For this review, take the finished solid that the model builds, in its own axes (mm). A direction names the side the tool comes from. Coordinates: 2 decimals unless noted, no trailing zeros. One line per item, written item: value.
from build123d import *

# Parameters (mm, degrees)
ESQUISSE1_R                  = 8
BOSS_EXTRU_1_DEPTH           = 16
ENL_V_MAT_EXTRU_1_DEPTH      = 10
ESQUISSE3_R                  = 5
ENL_V_MAT_EXTRU_2_DEPTH      = 20.595917942
R_P_TITION_CIRCULAIRE1_COUNT = 10
CONG_1_R                     = 1
CONG_2_R                     = 1
BOSS_EXTRU_2_DEPTH           = 2
ESQUISSE5_R                  = 3.4
ENL_V_MAT_EXTRU_3_DEPTH      = 3.5
ESQUISSE6_R                  = 0.5
ENL_V_MAT_EXTRU_4_DEPTH      = 6.5
CONG_3_R                     = 2


# Some blends are built 0.0001 mm under size
with BuildPart() as part:
    # Esquisse1 → Boss.-Extru.1 (new body)
    with BuildSketch(Plane(origin=(0, 0, 0), x_dir=(1, 0, 0), z_dir=(0, 1, 0))):
        with Locations(Location((0, 0, 0), (0, 0, 270))):
            Circle(ESQUISSE1_R)
    extrude(amount=BOSS_EXTRU_1_DEPTH)

    # Esquisse2 → Enlèv. mat.-Extru.1 (cut)
    with BuildSketch(Plane(origin=(0, 16, 0), x_dir=(1, 0, 0), z_dir=(0, 1, 0))):
        with BuildLine():
            ThreePointArc((0, 3.15), (-2.720753572, 1.587450787), (-2.74226184, -1.55))
            Line((-2.74226184, -1.55), (0, -1.55))
            Line((0, -1.55), (0, 3.15))
        make_face()
        with BuildLine():
            Line((0, 3.15), (0, -1.55))
            Line((0, -1.55), (2.74226184, -1.55))
            ThreePointArc((2.74226184, -1.55), (3.046360517, -0.801366085), (3.15, 0))
            ThreePointArc((3.15, 0), (2.227386361, 2.227386361), (0, 3.15))
        make_face()
    extrude(amount=-ENL_V_MAT_EXTRU_1_DEPTH, mode=Mode.SUBTRACT)

    # Esquisse3 → Enlèv. mat.-Extru.2 (cut, through all)
    with BuildSketch(Plane(origin=(0, 16, 0), x_dir=(1, 0, 0), z_dir=(0, 1, 0))):
        with Locations((0, 12.5)):
            Circle(ESQUISSE3_R)
    enl_v_mat_extru_2 = extrude(amount=-ENL_V_MAT_EXTRU_2_DEPTH, mode=Mode.SUBTRACT)

    # Répétition circulaire1: Enlèv. mat.-Extru.2 ×10 about axis
    r_p_tition_circulaire1_axis = Axis((0, 0, 0), (0, 1, 0))
    for i in range(1, R_P_TITION_CIRCULAIRE1_COUNT):
        add(enl_v_mat_extru_2.rotate(r_p_tition_circulaire1_axis, i * 360 / R_P_TITION_CIRCULAIRE1_COUNT), mode=Mode.SUBTRACT)

    # Congé1
    cong_1_edges = [part.edges().sort_by_distance(p)[0] for p in [
        (1.733176275, 8, -7.81),
        (-1.733176275, 8, -7.81),
        (-3.18843376, 8, -7.33715818),
        (-5.992771881, 8, -5.299687272),
        (-6.892170469, 8, -4.061771316),
        (-7.963332315, 8, -0.765074136),
        (-1.733176275, 8, 7.81),
        (1.733176275, 8, 7.81),
        (-7.963332315, 8, 0.765074136),
        (-6.892170469, 8, 4.061771316),
        (-5.992771881, 8, 5.299687272),
        (-3.18843376, 8, 7.33715818),
        (3.18843376, 8, 7.33715818),
        (5.992771881, 8, 5.299687272),
        (6.892170469, 8, 4.061771316),
        (7.963332315, 8, 0.765074136),
        (7.963332315, 8, -0.765074136),
        (6.892170469, 8, -4.061771316),
        (5.992771881, 8, -5.299687272),
        (3.18843376, 8, -7.33715818),
    ]]
    fillet(cong_1_edges, radius=CONG_1_R)

    # Congé2
    cong_2_edges = [part.edges().sort_by_distance(p)[0] for p in [
        (-2.472135955, 0, -7.60845213),
        (-6.472135955, 0, -4.702282018),
        (-4.408389392, 0, -6.067627458),
        (0, 0, -7.5),
        (2.472135955, 0, -7.60845213),
        (4.408389392, 0, -6.067627458),
        (6.472135955, 0, -4.702282018),
        (7.132923872, 0, -2.317627458),
        (8, 0, 0),
        (7.132923872, 0, 2.317627458),
        (6.472135955, 0, 4.702282018),
        (4.408389392, 0, 6.067627458),
        (2.472135955, 0, 7.60845213),
        (0, 0, 7.5),
        (-2.472135955, 0, 7.60845213),
        (-4.408389392, 0, 6.067627458),
        (-6.472135955, 0, 4.702282018),
        (-7.132923872, 0, 2.317627458),
        (-8, 0, 0),
        (-7.132923872, 0, -2.317627458),
        (-6.846351136, 0, -4.072559992),
        (-5.988873569, 0, -5.252776613),
        (-3.145023717, 0, -7.318954474),
        (-7.932605121, 0, -0.729413986),
        (-7.932605121, 0, 0.729413986),
        (-6.846351136, 0, 4.072559992),
        (-5.988873569, 0, 5.252776613),
        (-3.145023717, 0, 7.318954474),
        (-1.757595867, 0, 7.769757109),
        (1.757595867, 0, 7.769757109),
        (3.145023717, 0, 7.318954474),
        (5.988873569, 0, 5.252776613),
        (6.846351136, 0, 4.072559992),
        (7.932605121, 0, 0.729413986),
        (7.932605121, 0, -0.729413986),
        (6.846351136, 0, -4.072559992),
        (5.988873569, 0, -5.252776613),
        (3.145023717, 0, -7.318954474),
        (1.757595867, 0, -7.769757109),
        (-1.757595867, 0, -7.769757109),
    ]]
    fillet(cong_2_edges, radius=CONG_2_R - 0.0001)  # a hair under: the kernel refuses the full size

    # Esquisse4 → Boss.-Extru.2 (add)
    with BuildSketch(Plane(origin=(0, 16, 0), x_dir=(1, 0, 0), z_dir=(0, 1, 0))):
        with BuildLine():
            ThreePointArc((-1.483028995, 7.725), (0, 7.5), (1.483028995, 7.725))
            ThreePointArc((1.483028995, 7.725), (1.757595867, 7.769757113), (2.033868336, 7.737142857))
            ThreePointArc((2.033868336, 7.737142857), (2.472135955, 7.60845213), (2.902344418, 7.454957872))
            ThreePointArc((2.902344418, 7.454957872), (3.145023719, 7.318954477), (3.340845414, 7.121358854))
            ThreePointArc((3.340845414, 7.121358854), (4.408389392, 6.067627458), (5.740436734, 5.37795371))
            ThreePointArc((5.740436734, 5.37795371), (5.988873571, 5.252776617), (6.193212514, 5.064002246))
            ThreePointArc((6.193212514, 5.064002246), (6.472135955, 4.702282018), (6.729960252, 4.325232365))
            ThreePointArc((6.729960252, 4.325232365), (6.84635114, 4.072559993), (6.888630426, 3.797600671))
            ThreePointArc((6.888630426, 3.797600671), (7.132923872, 2.317627458), (7.805192751, 0.976711892))
            ThreePointArc((7.805192751, 0.976711892), (7.932605125, 0.729413987), (7.986960012, 0.456584897))
            ThreePointArc((7.986960012, 0.456584897), (8, 0), (7.986960012, -0.456584897))
            ThreePointArc((7.986960012, -0.456584897), (7.932605125, -0.729413987), (7.805192751, -0.976711892))
            ThreePointArc((7.805192751, -0.976711892), (7.132923872, -2.317627458), (6.888630426, -3.797600671))
            ThreePointArc((6.888630426, -3.797600671), (6.84635114, -4.072559993), (6.729960252, -4.325232365))
            ThreePointArc((6.729960252, -4.325232365), (6.472135955, -4.702282018), (6.193212514, -5.064002246))
            ThreePointArc((6.193212514, -5.064002246), (5.988873571, -5.252776617), (5.740436734, -5.37795371))
            ThreePointArc((5.740436734, -5.37795371), (4.408389392, -6.067627458), (3.340845414, -7.121358854))
            ThreePointArc((3.340845414, -7.121358854), (3.145023719, -7.318954477), (2.902344418, -7.454957872))
            ThreePointArc((2.902344418, -7.454957872), (2.472135955, -7.60845213), (2.033868336, -7.737142857))
            ThreePointArc((2.033868336, -7.737142857), (1.757595867, -7.769757113), (1.483028995, -7.725))
            ThreePointArc((1.483028995, -7.725), (0, -7.5), (-1.483028995, -7.725))
            ThreePointArc((-1.483028995, -7.725), (-1.757595867, -7.769757113), (-2.033868336, -7.737142857))
            ThreePointArc((-2.033868336, -7.737142857), (-2.472135955, -7.60845213), (-2.902344418, -7.454957872))
            ThreePointArc((-2.902344418, -7.454957872), (-3.145023719, -7.318954477), (-3.340845414, -7.121358854))
            ThreePointArc((-3.340845414, -7.121358854), (-4.408389392, -6.067627458), (-5.740436734, -5.37795371))
            ThreePointArc((-5.740436734, -5.37795371), (-5.988873571, -5.252776617), (-6.193212514, -5.064002246))
            ThreePointArc((-6.193212514, -5.064002246), (-6.472135955, -4.702282018), (-6.729960252, -4.325232365))
            ThreePointArc((-6.729960252, -4.325232365), (-6.84635114, -4.072559993), (-6.888630426, -3.797600671))
            ThreePointArc((-6.888630426, -3.797600671), (-7.132923872, -2.317627458), (-7.805192751, -0.976711892))
            ThreePointArc((-7.805192751, -0.976711892), (-7.932605125, -0.729413987), (-7.986960012, -0.456584897))
            ThreePointArc((-7.986960012, -0.456584897), (-8, 0), (-7.986960012, 0.456584897))
            ThreePointArc((-7.986960012, 0.456584897), (-7.932605125, 0.729413987), (-7.805192751, 0.976711892))
            ThreePointArc((-7.805192751, 0.976711892), (-7.132923872, 2.317627458), (-6.888630426, 3.797600671))
            ThreePointArc((-6.888630426, 3.797600671), (-6.84635114, 4.072559993), (-6.729960252, 4.325232365))
            ThreePointArc((-6.729960252, 4.325232365), (-6.472135955, 4.702282018), (-6.193212514, 5.064002246))
            ThreePointArc((-6.193212514, 5.064002246), (-5.988873571, 5.252776617), (-5.740436734, 5.37795371))
            ThreePointArc((-5.740436734, 5.37795371), (-4.408389392, 6.067627458), (-3.340845414, 7.121358854))
            ThreePointArc((-3.340845414, 7.121358854), (-3.145023719, 7.318954477), (-2.902344418, 7.454957872))
            ThreePointArc((-2.902344418, 7.454957872), (-2.472135955, 7.60845213), (-2.033868336, 7.737142857))
            ThreePointArc((-2.033868336, 7.737142857), (-1.757595867, 7.769757113), (-1.483028995, 7.725))
        make_face()
        with BuildLine():
            ThreePointArc((-6.98859001, 0.399511784), (-6.181867356, 2.008610463), (-5.88871522, 3.784578319))
            ThreePointArc((-5.88871522, 3.784578319), (-5.663118961, 4.114496766), (-5.41906095, 4.431001966))
            ThreePointArc((-5.41906095, 4.431001966), (-3.82060414, 5.258610463), (-2.539551366, 6.523088138))
            ThreePointArc((-2.539551366, 6.523088138), (-2.163118961, 6.657395614), (-1.779634794, 6.77))
            ThreePointArc((-1.779634794, 6.77), (0, 6.5), (1.779634794, 6.77))
            ThreePointArc((1.779634794, 6.77), (2.163118961, 6.657395614), (2.539551366, 6.523088138))
            ThreePointArc((2.539551366, 6.523088138), (3.82060414, 5.258610463), (5.41906095, 4.431001966))
            ThreePointArc((5.41906095, 4.431001966), (5.663118961, 4.114496766), (5.88871522, 3.784578319))
            ThreePointArc((5.88871522, 3.784578319), (6.181867356, 2.008610463), (6.98859001, 0.399511784))
            ThreePointArc((6.98859001, 0.399511784), (7, 0), (6.98859001, -0.399511784))
            ThreePointArc((6.98859001, -0.399511784), (6.181867356, -2.008610463), (5.88871522, -3.784578319))
            ThreePointArc((5.88871522, -3.784578319), (5.663118961, -4.114496766), (5.41906095, -4.431001966))
            ThreePointArc((5.41906095, -4.431001966), (3.82060414, -5.258610463), (2.539551366, -6.523088138))
            ThreePointArc((2.539551366, -6.523088138), (2.163118961, -6.657395614), (1.779634794, -6.77))
            ThreePointArc((1.779634794, -6.77), (0, -6.5), (-1.779634794, -6.77))
            ThreePointArc((-1.779634794, -6.77), (-2.163118961, -6.657395614), (-2.539551366, -6.523088138))
            ThreePointArc((-2.539551366, -6.523088138), (-3.82060414, -5.258610463), (-5.41906095, -4.431001966))
            ThreePointArc((-5.41906095, -4.431001966), (-5.663118961, -4.114496766), (-5.88871522, -3.784578319))
            ThreePointArc((-5.88871522, -3.784578319), (-6.181867356, -2.008610463), (-6.98859001, -0.399511784))
            ThreePointArc((-6.98859001, -0.399511784), (-7, 0), (-6.98859001, 0.399511784))
        make_face(mode=Mode.SUBTRACT)
    extrude(amount=BOSS_EXTRU_2_DEPTH)

    # Esquisse5 → Enlèv. mat.-Extru.3 (cut)
    with BuildSketch(Plane(origin=(0, 16, 0), x_dir=(1, 0, 0), z_dir=(0, 1, 0))):
        with Locations(Location((0, 0, 0), (0, 0, 270))):
            Circle(ESQUISSE5_R)
    extrude(amount=-ENL_V_MAT_EXTRU_3_DEPTH, mode=Mode.SUBTRACT)

    # Esquisse6 → Enlèv. mat.-Extru.4 (cut)
    with BuildSketch(Plane(origin=(0, 12.5, 0), x_dir=(1, 0, 0), z_dir=(0, 1, 0))):
        with Locations((0, -1.55)):
            Circle(ESQUISSE6_R)
    extrude(amount=-ENL_V_MAT_EXTRU_4_DEPTH, mode=Mode.SUBTRACT)

    # Congé3
    # the kernel refuses this fillet: 2 mm, written as the material it takes off along each edge
    with BuildSketch(Plane(origin=(-0.5, 6, 1.55), x_dir=(-1, 0, 0), z_dir=(0, 1, 0))) as cong_3_piece_1:
        with BuildLine():
            CenterArc((1, 2), CONG_3_R, 233.130102354, 36.869897646)
            ThreePointArc((-0.2, 0.4), (-0.052786405, 0.223606798), (0, 0))
            Line((0, 0), (1, 0))
        make_face()
    extrude(amount=9, mode=Mode.SUBTRACT)
    with BuildSketch(Plane(origin=(0.5, 15, 1.55), x_dir=(-0.4472135954998809, 0, 0.8944271909999544), z_dir=(0, -1, 0))) as cong_3_piece_2:
        with BuildLine():
            CenterArc((1.341640786, -1.788854382), CONG_3_R, 116.565051177, 36.869897646)
            Line((-0.447213596, -0.894427191), (0, 0))
            ThreePointArc((0, 0), (0.223606798, -0.052786405), (0.447213595, 0))
        make_face()
    extrude(amount=9, mode=Mode.SUBTRACT)


solid = part.part
1. To check wall thickness, follow probe 1 along X at (y, z) = (14.75, 0); probe 2 along X at (y, z) = (10.75, 3.75); probe 3 along Y at (x, z) = (-5, 2). State the ranges of each line that lie inside material, in increasing order. Write a range as from..to.
Return value:
probe 1: x = -8..-3.4, 3.4..8
probe 2: x = -6.89..6.89
probe 3: y = 0..16
2. The part is to be moulded in two halves that separate along Z. For faces 1 (the flat face through (4.2, 18, -5.2)), 2 (the cylindrical face through (0, 9.4, -7.5)), 3 (the cylindrical face through (0, 17, 6.5)), say which applies: pulls with the +Z half, pulls with the -Z half, needs draft (parallel to the pull), parting line crosses it, or undercut.
Return value:
face 1: needs draft
face 2: pulls with the -Z half
face 3: undercut
3. For faces 4 (the cylindrical face through (-3.8, 16.986, 5.274)), 5 (the cylindrical face through (0, 9.4, 7.5)), list the 3-axis set-ups (+Z, -Z, +X, -X, +Y, -Y) from which the entire face can be reached by the end or side of a thin tool; tool diameter is ignored.
Return value:
face 4: +Y
face 5: +Z, +Y, -Y
4. Insertion check: pin 1 Ø0.6 at (x, y) = (-2.5, 10.5) entering from -Z; pin 2 Ø2 at (x, z) = (-1.5, -1) entering from +Y; pin 3 Ø1 at (x, z) = (-4, -2) entering from +Y. Each pin has a flat end and moves straight along its axis. Give the tip position at first contact, or say it passes through.
Return value:
pin 1: stops at z = -7.69
pin 2: stops at y = 6
pin 3: stops at y = 16
